Can you work these out from the model? Positions are in its coordinate system, mm. A direction names the side the tool comes from. Round coordinates to 2 decimals unless told otherwise and drop trailing zeros. Order: outer loops, then holes, each group sorted by start corner. A loop starts at its lowest first (then second) coordinate and runs counter-clockwise, first axis right, second up.
Q1. Will these pins go through, and if not, where does the flat tip stop? P1, Ø3.5, axis at x = 15.53, y = 102.96, coming from the +Z side; P2, Ø1.5, axis at y = 38, z = 7, coming from the +X side; P3, Ø4, axis at y = 68, z = 7.5, coming from the -X side.
Q2. We'd pull the mould along Y, two halves only. Please class faces 3 (the face through (3.044, 75.678, 4.807)), 4 (the face through (15.262, 104.988, 4.807)), 5 (the face through (-0.267, 47.033, 4.807)), 6 (the face through (12.745, 73.245, 4.807)): pulls with the +Y half, pulls with the -Y half, needs draft (parallel to the pull), parting line crosses it, or undercut.
Q3. If we section it at D-D (x = 7.25): Please give me the cut outline in (y, z), plus the area to 3 significant figures.
Q4. If we section it at C-C (y = 36): Please give me the cut outline in (x, z), plus the area to 3 significant figures.
Q5. If we section it at A-A (z = 7.75): Please give me the cut outline in (x, y).
Q6. For faces 1 (the face through (-0.267, 2.033, 4.807)), 2 (the face through (5, 21, 5)), which set-ups out of +Z, -Z, +X, -X, +Y, -Y let a thin tool reach every point of the face, with its end or its side?
Q7. If we section it at B-B (x = 0): Please give me the cut outline in (y, z), plus the area to 3 significant figures.
Q8. If I drill on line 1 (X direction, y = 6, z = 8.5); line 2 (X direction, y = 99, z = 6.25), over which ranges is the centre line in solid material (lowest first)?
from build123d import *

# Parameters (mm, degrees)
ESQUISSE1_R        = 2.05
BOSS_EXTRU_1_DEPTH = 9.75
CONG_1_R           = 10


with BuildPart() as part:
    # Esquisse1 → Boss.-Extru.1 (new body)
    # profile 1 of 3: a face of its own
    with BuildSketch(Plane.XY):
        with BuildLine():
            Line((10.699513575, 104.249644803), (-4.829629131, 46.294095226))
            ThreePointArc((-4.829629131, 46.294095226), (0.652630961, 49.957224307), (5, 45))
            Line((5, 45), (5, 44.341737512))
            Line((5, 44.341737512), (20.358771838, 101.661454352))
            ThreePointArc((20.358771838, 101.661454352), (16.823237932, 107.785178709), (10.699513575, 104.249644803))
        make_face()
        with Locations((15.529142706, 102.955549577)):
            Circle(ESQUISSE1_R, mode=Mode.SUBTRACT)
    # profile 2 of 3: a face of its own
    with BuildSketch(Plane.XY):
        with BuildLine():
            ThreePointArc((-4.829629131, 46.294095226), (-4.957224307, 45.652630961), (-5, 45))
            ThreePointArc((-5, 45), (-0.652630961, 40.042775693), (4.829629131, 43.705904774))
            Line((4.829629131, 43.705904774), (5, 44.341737512))
            Line((5, 44.341737512), (5, 45))
            ThreePointArc((5, 45), (0.652630961, 49.957224307), (-4.829629131, 46.294095226))
        make_face()
        with Locations((0, 45)):
            Circle(ESQUISSE1_R, mode=Mode.SUBTRACT)
    # profile 3 of 3: a face of its own
    with BuildSketch(Plane.XY):
        with BuildLine():
            Line((-5, 45), (-5, 0))
            ThreePointArc((-5, 0), (0, -5), (5, 0))
            Line((5, 0), (5, 44.341737512))
            Line((5, 44.341737512), (4.829629131, 43.705904774))
            ThreePointArc((4.829629131, 43.705904774), (-0.652630961, 40.042775693), (-5, 45))
        make_face()
        Circle(ESQUISSE1_R, mode=Mode.SUBTRACT)
    extrude(amount=BOSS_EXTRU_1_DEPTH)

    # Congé1
    cong_1_edges = [part.edges().sort_by_distance(p)[0] for p in [
        (5, 44.341737512, 4.875),
    ]]
    fillet(cong_1_edges, radius=CONG_1_R)


solid = part.part
Solution:
1. P1: passes through
1. P2: stops at x = 5
1. P3: stops at x = 0.45
2. face 3: pulls with the +Y half
2. face 4: undercut
2. face 5: undercut
2. face 6: pulls with the -Y half
3. outline: (52.74, 0) - (91.38, 0) - (91.38, 9.75) - (52.74, 9.75) - close
3. area: 377 mm2
4. outline: (-5, 0) - (5, 0) - (5, 9.75) - (-5, 9.75) - close
4. area: 97.5 mm2
5. outline: (-5, 0) arc R5 ccw to (5, 0) - (5, 43.03) arc R10 cw to (5.34, 45.61) - (20.36, 101.66) arc R5 ccw to (10.7, 104.25) - (-4.83, 46.29) arc R5 ccw to (-5, 45) - close; hole circle Ø4.1 at (0, 0); hole circle Ø4.1 at (0, 45); hole circle Ø4.1 at (15.53, 102.96)
6. face 1: +Z, -Z
6. face 2: +Z, -Z, +X, -Y
7. outline: (-5, 0) - (-2.05, 0) - (-2.05, 9.75) - (-5, 9.75) - close; (2.05, 0) - (42.95, 0) - (42.95, 9.75) - (2.05, 9.75) - close; (47.05, 0) - (64.32, 0) - (64.32, 9.75) - (47.05, 9.75) - close
7. area: 596 mm2
8. line 1: x = -5 to 5
8. line 2: x = 9.29 to 19.65
